For this review, take the finished solid that the model builds, in its own axes (mm). Give positions to 0.01 mm unless a question says otherwise; leave off trailing zeros. Write each loop counter-clockwise with the first axis right and the second up, starting at its lowest first coordinate (ties: lowest second). Pieces come first, ordered by that corner, then holes. Notation, with made-up numbers: (18, -35.5) -> (33, -35.5) arc R28 cw to (33, -6.5) -> close; hole circle Ø11 at (63.5, 71.25). An arc over 180 degrees is marked (long way). Write item = value, one per line.
```python
from build123d import *

# Parameters (mm, degrees)
SKETCH_1_R      = 28
SKETCH_1_R_2    = 7
EXTRUDE_1_DEPTH = 25


with BuildPart() as part:
    # 草图1 → 凸台-拉伸1 (new body)
    with BuildSketch(Plane(origin=(0, 0, 0), x_dir=(1, 0, 0), z_dir=(0, 1, 0))):
        with BuildLine():
            Line((180, 28), (-180, 28))
            ThreePointArc((-180, 28), (-160.201010127, 19.798989873), (-152, 0))
            ThreePointArc((-152, 0), (-160.201010127, -19.798989873), (-180, -28))
            Line((-180, -28), (180, -28))
            ThreePointArc((180, -28), (152, 0), (180, 28))
        make_face()
        with Locations((180, 0)):
            Circle(SKETCH_1_R)
        with Locations((180, 0)):
            Circle(SKETCH_1_R_2, mode=Mode.SUBTRACT)
        with Locations((-180, 0)):
            Circle(SKETCH_1_R)
        with Locations((-180, 0)):
            Circle(SKETCH_1_R_2, mode=Mode.SUBTRACT)
    extrude(amount=EXTRUDE_1_DEPTH)


solid = part.part
```
(1) Take a section at A-A (z = 0). Write out the cut boundary in (x, y), plus the area to 3 significant figures.
Answers below:
outline = (-208, 0) -> (-187, 0) -> (-187, 25) -> (-208, 25) -> close; (-173, 0) -> (173, 0) -> (173, 25) -> (-173, 25) -> close; (187, 0) -> (208, 0) -> (208, 25) -> (187, 25) -> close
area = 9,700 mm^2
(2) Take a section at B-B (y = 7). Write out the cut boundary in (x, z), plus the area to 3 significant figures.
Answers below:
outline = (-180, -28) -> (180, -28) arc R28 ccw to (180, 28) -> (-180, 28) arc R28 ccw to start; hole circle Ø14 at (-180, 0); hole circle Ø14 at (180, 0)
area = 22,300 mm^2
(3) The part is to be moulded in two halves that separate along Z. For faces 1 (the face through (3, 12, -28)), 2 (the face through (-3, 0, 0)), 3 (the face through (-173.534, 12.325, 2.681)), say which applies: released by +Z, released by -Z, zero draft, split by the parting line, or undercut.
Answers below:
face_1 = released by -Z
face_2 = zero draft
face_3 = undercut
(4) To check wall thickness, follow probe 1 along X at (y, z) = (10.25, 0); probe 2 along Z at (x, y) = (180, 10.5); probe 3 along X at (y, z) = (14.75, 5.5). State the ranges of each line that lie inside material, in increasing order.
Answers below:
probe_1 = -208 to -187, -173 to 173, 187 to 208
probe_2 = -28 to -7, 7 to 28
probe_3 = -207.45 to -184.33, -175.67 to 175.67, 184.33 to 207.45
(5) For pin 1 (5 mm diameter, centred on y = 21, z = -12, fed in from +X); pin 2 (11 mm diameter, centred on x = -180, z = 0, fed in from +Y); pin 3 (1 mm diameter, centred on y = 4, z = 10.5, fed in from -X); pin 4 (10 mm diameter, centred on y = 19, z = 13.5, fed in from -X), all flat-tipped, find the tip position at first contact; note any pin that passes through.
Answers below:
pin_1 = 206.34
pin_2 = through
pin_3 = -206.15
pin_4 = -206.68
(6) Take a section at C-C (z = -22.5). Write out the cut boundary in (x, y), plus the area to 3 significant figures.
Answers below:
outline = (-196.67, 0) -> (196.67, 0) -> (196.67, 25) -> (-196.67, 25) -> close
area = 9,830 mm^2
